from build123d import *

# Parameters (mm, degrees)
SKETCH1_R                  = 31.75
BOSS_EXTRUDE1_DEPTH        = 34.925
SKETCH3_R                  = 25.4
BOSS_EXTRUDE2_DEPTH        = 38.1
F_97_1_DIAMETER_HOLE1_D    = 25.4
F_97_1_25_DIAMETER_HOLE1_D = 31.75


with BuildPart() as part:
    # Sketch1 → Boss-Extrude1 (new body, symmetric)
    with BuildSketch(Plane.XY):
        with BuildLine():
            ThreePointArc((-31.75, 0), (0, 31.75), (31.75, 0))
            Line((31.75, 0), (31.75, 69.85))
            Line((31.75, 69.85), (-31.75, 69.85))
            Line((-31.75, 69.85), (-31.75, 0))
        make_face()
        Circle(SKETCH1_R)
    extrude(amount=BOSS_EXTRUDE1_DEPTH, both=True)

    # Sketch3 → Boss-Extrude2 (add, symmetric)
    with BuildSketch(Plane(origin=(0, 0, 0), x_dir=(0, 0, -1), z_dir=(1, 0, 0))):
        with Locations((0, 69.85)):
            Circle(SKETCH3_R)
    extrude(amount=BOSS_EXTRUDE2_DEPTH, both=True)

    # #97 (1) Diameter Hole1 (through all)
    with Locations(Plane(origin=(38.1, 0, 0), x_dir=(0, 0, -1), z_dir=(1, 0, 0))):
        with Locations((0, 69.85)):
            Hole(F_97_1_DIAMETER_HOLE1_D / 2)

    # #97 (1.25) Diameter Hole1 (through all)
    with Locations(Plane(origin=(0, 0, -34.925), x_dir=(-1, 0, 0), z_dir=(0, 0, -1))):
        with Locations((0, 0)):
            Hole(F_97_1_25_DIAMETER_HOLE1_D / 2)


solid = part.part
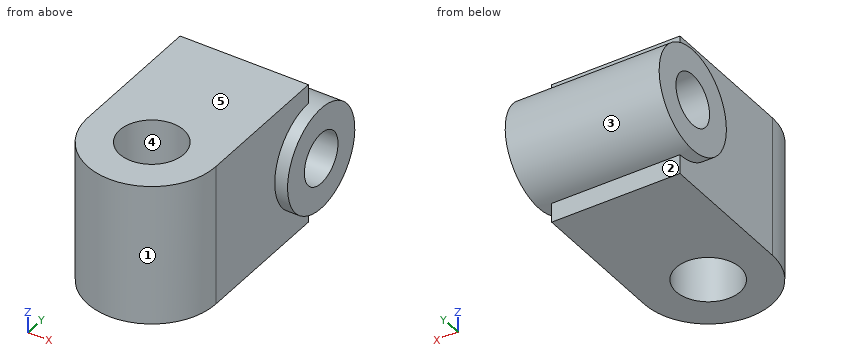
Build history of the part. All positions in model axes, mm. Face numbers are marked on the shaded views. A direction names the side the tool comes from. Round coordinates to 2 decimals unless told otherwise and drop trailing zeros. Loops run counter-clockwise (first coordinate to the right, second up) from the corner with the lowest first, then second, coordinate; pieces in that order, holes last. Notation, with made-up numbers: (-34.75, 50.5) -> (4.25, 50.5) arc R23 ccw to (4.25, 83.5) -> close; hole circle Ø11 at (49, 50.25). An arc over 180 degrees is marked (long way). One line per item, written item: value. Start each with the question number.
Q1. 3-axis set-ups, long thin cutter, end or side, ignore diameter. For the marked faces 1 and 2: which of +Z, -Z, +X, -X, +Y, -Y reach the whole face in a straight line?
Q2. Cut at A-A on z = 0. List the corners of the cut face in (x, y) (3 decimals), plus the area to 3 significant figures.
Q3. Two-plate mould, pull along Y, no slides. Class the marked faces 3, 4 and 5: released by +Y, released by -Y, zero draft, split by the parting line, or undercut.
Q4. Cut at C-C on y = 80. List the corners of the cut face in (x, z), plus the area to 3 significant figures.
Q5. Probe line 1 along Y through (x, z) = (0, 0) (3 decimals); line 2 along Z through (x, y) = (-23.5, 70); line 3 along X through (y, z) = (25.5, -9). List the from-to ranges inside material, lowest first.
Q6. Cut at D-D on x = 25. List the corners of the cut face in (y, z) (3 decimals), plus the area to 3 significant figures.
Q7. Cut at B-B on x = 0. List the corners of the cut face in (y, z) (3 decimals), plus the area to 3 significant figures.
Q8. Drop flat-ended pins along their axis: pin 1 Ø5 at (x, z) = (-4, 31.5) entering from +Y; pin 2 Ø1.5 at (x, z) = (-6.5, 11.5) entering from -Y (3 decimals); pin 3 Ø15 at (y, z) = (69.85, 0) entering from +X; pin 4 Ø12 at (x, z) = (7.5, 1.5) entering from -Y. Give the stop position or say it passes through.
Computed:
1. face 1: +Z, -Z, -Y
1. face 2: -Z, +X, -X, +Y
2. outline: (-38.1, 44.45) -> (-31.75, 44.45) -> (-31.75, 0) arc R31.75 ccw to (31.75, 0) -> (31.75, 44.45) -> (38.1, 44.45) -> (38.1, 57.15) -> (-38.1, 57.15) -> close; (-38.1, 82.55) -> (38.1, 82.55) -> (38.1, 95.25) -> (-38.1, 95.25) -> close; hole circle Ø31.75 at (0, 0)
2. area: 5,550 mm²
3. face 3: split by the parting line
3. face 4: undercut
3. face 5: zero draft
4. outline: (-38.1, -23.28) -> (38.1, -23.28) -> (38.1, -7.63) -> (-38.1, -7.63) -> close; (-38.1, 7.63) -> (38.1, 7.63) -> (38.1, 23.28) -> (-38.1, 23.28) -> close
4. area: 2,390 mm²
5. line 1: -31.75 to -15.875, 15.875 to 57.15, 82.55 to 95.25
5. line 2: -25.4 to -12.7, 12.7 to 25.4
5. line 3: -31.75 to 31.75
6. outline: (-19.572, -34.925) -> (69.85, -34.925) -> (69.85, -25.4) arc R25.4 ccw to (69.85, 25.4) -> (69.85, 34.925) -> (-19.572, 34.925) -> close; hole circle Ø25.4 at (69.85, 0)
6. area: 6,750 mm²
7. outline: (-31.75, -34.925) -> (-15.875, -34.925) -> (-15.875, 34.925) -> (-31.75, 34.925) -> close; (15.875, -34.925) -> (69.85, -34.925) -> (69.85, -25.4) arc R25.4 ccw to (69.85, 25.4) -> (69.85, 34.925) -> (15.875, 34.925) -> close; hole circle Ø25.4 at (69.85, 0)
7. area: 5,390 mm²
8. pin 1: y = 69.85
8. pin 2: y = -31.225
8. pin 3: through
8. pin 4: y = -31.71
